Autodesk Inventor part; units mm, degrees
ref_plane "YZ Plane" through (0, 0, 0) normal (1, 0, 0) x (0, 1, 0)
ref_plane "XZ Plane" through (0, 0, 0) normal (0, 1, 0) x (-1, 0, 0)
ref_plane "XY Plane" through (0, 0, 0) normal (0, 0, 1) x (1, 0, 0)
sketch "Boceto1" plane through (0, 0, 0) normal (0, 1, 0) x (-1, 0, 0)
  line L0 (0, 0) -> (10.9, 0)
  line L1 (10.9, 0) -> (10.9, 24)
  line L2 (10.9, 31) -> (0, 31)
  line L3 (0, 24) -> (0, 0)
  line L4 (10.9, 31) -> (10.4, 31)
  line L5 (15.4, 26) -> (15.4, 26)
  line L6 (15.4, 26) -> (12.9, 26)
  line L7 (10.9, 26) -> (10.9, 31)
  line L8 (0, 31) -> (0.5, 31)
  line L9 (-4.5, 26) -> (-4.5, 26)
  line L10 (-4.5, 26) -> (-2, 26)
  line L11 (0, 26) -> (0, 31)
  arc A0 (15.4, 26) -> (10.4, 31) centre (10.4, 26) ccw
  arc A1 (0.5, 31) -> (-4.5, 26) centre (0.5, 26) ccw
  arc A2 (12.9, 26) -> (10.9, 24) centre (12.9, 24) ccw
  arc A3 (0, 24) -> (-2, 26) centre (-2, 24) ccw
  point P0 (15.4, 31)
  point P1 (-4.5, 31)
  dimension "d0" = 10.9
  dimension "d1" = 31
  dimension "d2" = 4.5
  dimension "d3" = 5
  dimension "d4" = 4.5
  dimension "d5" = 5
  dimension "d7" = 5
  dimension "d8" = 5
  dimension "d9" = 2
extrude "Extrusión1" add sketch "Boceto1" along normal blind 4.5 contours L3 A3 L10 A1 L2 A0 L6 A2 L1 L0
sketch "Boceto2" plane through (0, 4.5, 0) normal (0, 1, 0) x (1, 0, 0)
  arc A0 (-15.4, -26) -> (-10.4, -31) centre (-10.4, -26) ccw
  line L0 (-10.4, -31) -> (-0.5, -31)
  arc A1 (-0.5, -31) -> (4.5, -26) centre (-0.5, -26) ccw
  line L1 (4.5, -26) -> (2, -26)
  arc A2 (0, -24) -> (2, -26) centre (2, -24) ccw
  line L2 (0, -24) -> (0, 0)
  line L3 (0, 0) -> (-10.9, 0)
  line L4 (-10.9, 0) -> (-10.9, -24)
  arc A3 (-12.9, -26) -> (-10.9, -24) centre (-12.9, -24) ccw
  line L5 (-12.9, -26) -> (-15.4, -26)
  line L6 (-9.05, -24) -> (-9.05, -1.85)
  line L7 (-9.05, -1.85) -> (-1.85, -1.85)
  line L8 (-1.85, -1.85) -> (-1.85, -24)
  arc A4 (-1.85, -24) -> (2, -27.85) centre (2, -24) ccw
  line L9 (2, -27.85) -> (2.0495, -27.85)
  arc A5 (-0.5, -29.15) -> (2.0495, -27.85) centre (-0.5, -26) ccw
  line L10 (-0.5, -29.15) -> (-10.4, -29.15)
  arc A6 (-12.9495, -27.85) -> (-10.4, -29.15) centre (-10.4, -26) ccw
  line L11 (-12.9495, -27.85) -> (-12.9, -27.85)
  arc A7 (-12.9, -27.85) -> (-9.05, -24) centre (-12.9, -24) ccw
  line L12 (-5.45, -1.85) -> (-5.45, -15.85)
  line L13 (-5.45, -15.85) -> (-9.05, -15.85)
  line L14 (-5.45, -15.85) -> (-1.85, -15.85)
  dimension "d14" = 7.2
  dimension "d15" = 14
extrude "Extrusión2" cut sketch "Boceto2" against normal blind 3 contours L6 L7 L12 L13 | L12 L7 L8 L14
sketch "Boceto3" plane through (0, 1.5, 0) normal (0, 1, 0) x (1, 0, 0)
  line L0 (-1.85, -1.85) -> (-1.85, -15.85)
  line L1 (-9.05, -1.85) -> (-1.85, -1.85)
  line L2 (-9.05, -15.85) -> (-9.05, -1.85)
  line L3 (-1.85, -15.85) -> (-9.05, -15.85)
  line L4 (-5.45, -3.4) -> (-5.45, -3.4)
  line L5 (-3.4, -5.45) -> (-3.4, -12.25)
  line L6 (-5.45, -14.3) -> (-5.45, -14.3)
  line L7 (-7.5, -12.25) -> (-7.5, -5.45)
  arc A0 (-5.45, -3.4) -> (-7.5, -5.45) centre (-5.45, -5.45) ccw
  arc A1 (-5.45, -14.3) -> (-3.4, -12.25) centre (-5.45, -12.25) ccw
  arc A2 (-7.5, -12.25) -> (-5.45, -14.3) centre (-5.45, -12.25) ccw
  arc A3 (-3.4, -5.45) -> (-5.45, -3.4) centre (-5.45, -5.45) ccw
  point P0 (0, 0)
  dimension "d18" = 4.1
  dimension "d19" = 2.05
extrude "Extrusión3" cut sketch "Boceto3" against normal blind 3 contours L5 A1 A2 L7 A0 A3
fillet "Empalme1" radius 0.5 4 edges at (0, 2.25, 0) (-10.9, 2.25, 0) (4.5, 2.25, 26) (-15.4, 2.25, 26)
properties part number "Cierre ventanas"
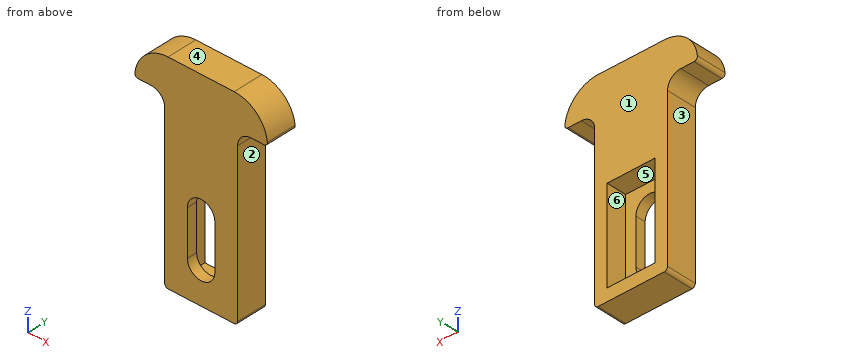
Design review of the part built by this model. Coordinates are the model's own, in mm. Face numbers are marked on the shaded views. A direction names the side the tool comes from. Coordinates: 2 decimals unless noted, no trailing zeros. Order: outer loops, then holes, each group sorted by start corner. A loop starts at its lowest first (then second) coordinate and runs counter-clockwise, first axis right, second up. Notation, with made-up numbers: M 62.25,4.25 L 106.25,4.25 A16 cw 106.25,34.25 Z; hole C 89,24 d10. An arc over 180 degrees is marked long. Use a Markdown table: item, result.
(1) Add section C-C (y = 4.2). Give the boundary of the cut face in (x, z).
Worked answers:
| item | result |
|---|---|
| outline | M -15.37,26.56 A0.5 ccw -14.87,26 L -12.9,26 A2 cw -10.9,24 L -10.9,0.5 A0.5 ccw -10.4,0 L -0.5,0 A0.5 ccw 0,0.5 L 0,24 A2 cw 2,26 L 3.97,26 A0.5 ccw 4.47,26.56 A5 ccw -0.5,31 L -10.4,31 A5 ccw Z; hole M -9.05,1.85 L -1.85,1.85 L -1.85,15.85 L -9.05,15.85 Z |
(2) Add section D-D (z = 3). Give the boundary of the cut face in (x, y).
Worked answers:
| item | result |
|---|---|
| outline | M -10.9,0 L 0,0 L 0,4.5 L -1.85,4.5 L -1.85,1.5 L -9.05,1.5 L -9.05,4.5 L -10.9,4.5 Z |
(3) Add section B-B (z = 11.5). Give the boundary of the cut face in (x, y), then the cut area to 3 significant figures.
Worked answers:
| item | result |
|---|---|
| outline | M -10.9,0 L -7.5,0 L -7.5,1.5 L -9.05,1.5 L -9.05,4.5 L -10.9,4.5 Z; M -3.4,0 L 0,0 L 0,4.5 L -1.85,4.5 L -1.85,1.5 L -3.4,1.5 Z |
| area | 21.3 mm2 |
(4) Draft analysis for pull direction Z (two halves, no side actions). For the marked faces 3, 4, 5 and 6, state which applies: released by +Z, released by -Z, zero draft, split by the parting line, or undercut.
Worked answers:
| item | result |
|---|---|
| face 3 | zero draft |
| face 4 | released by +Z |
| face 5 | undercut |
| face 6 | undercut |
(5) Add section A-A (x = -5). Give the boundary of the cut face in (y, z), then the cut area to 3 significant figures.
Worked answers:
| item | result |
|---|---|
| outline | M 0,0 L 4.5,0 L 4.5,1.85 L 1.5,1.85 L 1.5,3.45 L 0,3.45 Z; M 0,14.25 L 1.5,14.25 L 1.5,15.85 L 4.5,15.85 L 4.5,31 L 0,31 Z |
| area | 81.3 mm2 |
(6) For P1, Ø8, axis at x = -5.5, z = 11, coming from the +Y side; P2, Ø1.5, axis at y = 0.5, z = 7, coming from the -X side; P3, Ø1, axis at x = -14, y = 3, coming from the -Z side; P4, Ø1.5, axis at y = 1.5, z = 5, coming from the +X side, all flat-tipped, find the tip position at first contact; note any pin that passes through.
Worked answers:
| item | result |
|---|---|
| P1 | stops at y = 4.5 |
| P2 | stops at x = -10.9 |
| P3 | stops at z = 26 |
| P4 | stops at x = 0 |
(7) For the marked faces 1 and 2, list the 3-axis set-ups (+Z, -Z, +X, -X, +Y, -Y) from which the entire face can be reached by the end or side of a thin tool; tool diameter is ignored.
Worked answers:
| item | result |
|---|---|
| face 1 | +Z, -Z, +X, -X, +Y |
| face 2 | -Z, +X, +Y, -Y |
(8) Wall thickness on probe 1 along Z at (x, y) = (-4.75, 3.25); probe 2 along X at (y, z) = (3.3, 7.5); probe 3 along X at (y, z) = (1.35, 10): over which ranges is each line inside the solid? List them lowest first.
Worked answers:
| item | result |
|---|---|
| probe 1 | z = 0 to 1.85, 15.85 to 31 |
| probe 2 | x = -10.9 to -9.05, -1.85 to 0 |
| probe 3 | x = -10.9 to -7.5, -3.4 to 0 |
